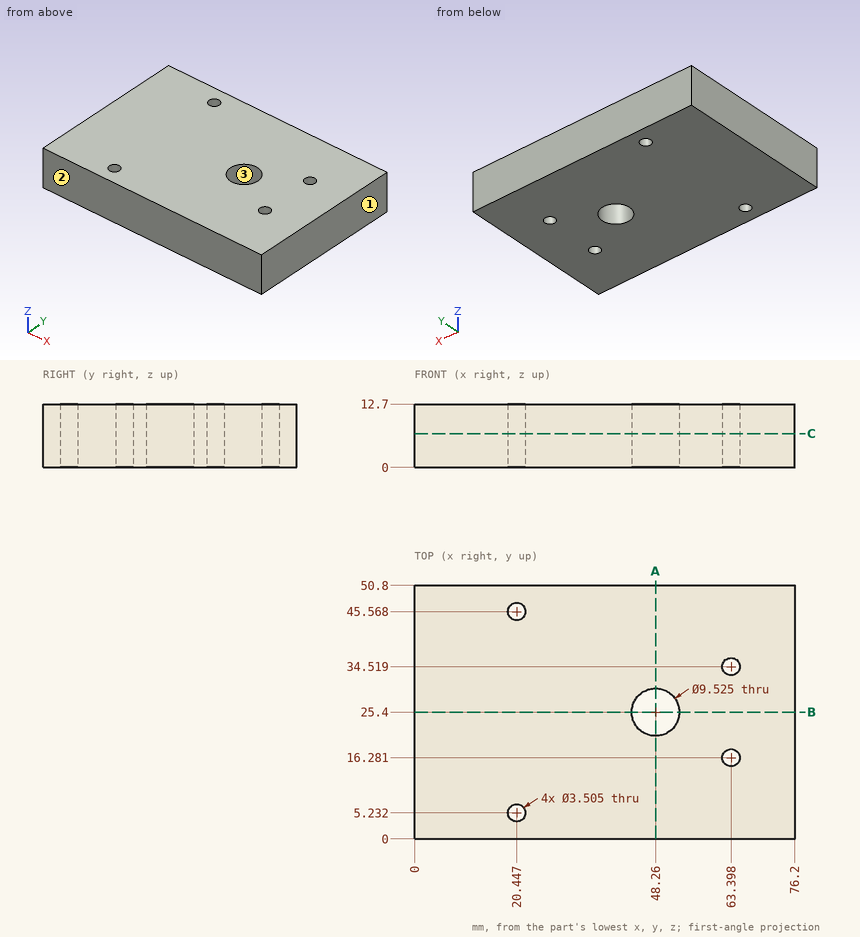
The figure shows three views and two pictorial views of one solid part (mm, origin at its lowest corner). Answer the questions. Give positions to 0.01 mm unless a question says otherwise; leave off trailing zeros. Write each loop counter-clockwise with the first axis right and the second up, starting at its lowest first coordinate (ties: lowest second). Pieces come first, ordered by that corner, then holes. Notation, with made-up numbers: M -17,37 L 39,37 A26 ccw 39,76 Z; hole C 10,-16.75 d4. An arc over 180 degrees is marked long. One line per item, written item: value. Start each with the question number.
(1) Find section A-A (x = 48.26). Determine the outline of the cut face in (y, z), plus the area to 3 significant figures.
(2) Find the intervals of material crossed by line 1 (Y direction, x = 63.5, z = 6); line 2 (Y direction, x = 65, z = 5.25) (1 decimal); line 3 (X direction, y = 6, z = 1.25), in increasing order.
(3) Find section B-B (y = 25.4). Determine the outline of the cut face in (x, z).
(4) Determine the mould class of the marked faces 1, 2 and 3 for opening direction X: pulls with the +X half, pulls with the -X half, needs draft (parallel to the pull), parting line crosses it, or undercut.
(5) A flat-ended cylindrical pin translates along its axis: pin 1 Ø3 at (x, y) = (63.4, 34.52) entering from -Z. Find the tip coordinate at first contact, or state that the pin passes through.
(6) Find section C-C (z = 6.75). Determine the outline of the cut face in (x, y) (1 decimal), plus the area to 3 significant figures.
Results below:
1. outline: M 0,0 L 20.64,0 L 20.64,12.7 L 0,12.7 Z; M 30.16,0 L 50.8,0 L 50.8,12.7 L 30.16,12.7 Z
1. area: 524 mm^2
2. line 1: y = 0 to 14.53, 18.03 to 32.77, 36.27 to 50.8
2. line 2: y = 0 to 15.6, 17 to 33.8, 35.2 to 50.8
2. line 3: x = 0 to 18.87, 22.02 to 76.2
3. outline: M 0,0 L 43.5,0 L 43.5,12.7 L 0,12.7 Z; M 53.02,0 L 76.2,0 L 76.2,12.7 L 53.02,12.7 Z
4. face 1: pulls with the +X half
4. face 2: needs draft
4. face 3: undercut
5. pin 1: passes through
6. outline: M 0,0 L 76.2,0 L 76.2,50.8 L 0,50.8 Z; hole C 20.4,5.2 d3.5; hole C 20.4,45.6 d3.5; hole C 48.3,25.4 d9.5; hole C 63.4,16.3 d3.5; hole C 63.4,34.5 d3.5
6. area: 3,760 mm^2
